Here's how the part is built. I have some questions about the finished solid (model axes, mm). A direction names the side the tool comes from. Coordinates: 2 decimals unless noted, no trailing zeros. Use one line per item in the form item = value. Start each with the question number.
(1) Will these pins go through, and if not, where does the flat tip stop? P1, Ø1.6, axis at x = 78, z = 74.5, coming from the -Y side; P2, Ø1.7, axis at x = 74.5, z = 139, coming from the +Y side; P3, Ø4, axis at y = 20, z = 222.5, coming from the -X side.
(2) Imagine slicing it at A-A, the plane y = 36. State how many separate pieces and enclosed holes the cut face has, and give its area (3 significant figures).
(3) Please list where these lines run through material, in increasing order: L1, parallel to Z at x = 196, y = 20; L2, parallel to Z at x = 45, y = 7; L3, parallel to X at y = 5.75, z = 74.5.
(4) On a 3-axis mill with a long thin cutter (end or side, diameter ignored), from which of +Z, -Z, +X, -X, +Y, -Y can I reach the whole of each face in a straight line? I mean faces 3 (the cylindrical face through (197.29, 17.52, 121.72)), 4 (the flat face through (124, 15, 121)). Say none if no direction works.
(5) Thinking about a two-plate mould opening in X: for faces 1 (the cylindrical face through (197.29, 17.52, 21.72)), 2 (the flat face through (195.455, 29.33, 120.785)), which applies, +X half, -X half, draft (parallel to the pull), parting line (faces both ways), or undercut?
```python
from build123d import *

# Parameters (mm, degrees)
EXTRUDE_1_DEPTH       = 245
EXTRUDE_3_DEPTH       = 245
PATTERN_CURVE_1_COUNT = 19
PATTERN_CURVE_1_PITCH = 9.75
SKETCH_6_R            = 2.5
CUT_EXTRUDE_3_DEPTH   = 8
SKETCH_7_R            = 2.6
CUT_EXTRUDE_4_DEPTH   = 6
SKETCH_8_R            = 4.5
SKETCH_8_R_2          = 3.4
CUT_EXTRUDE_5_DEPTH   = 6
CUT_EXTRUDE_START     = -6
SKETCH_9_R            = 2.6
CUT_EXTRUDE_6_DEPTH   = 6
EXTRUDE_4_REACH       = 321.453
SKETCH_11_R           = 2.6
EXTRUDE_5_REACH       = 321.453
SKETCH_12_R           = 4.5
SKETCH_12_R_2         = 3.4
SKETCH_19_R           = 2.6
CUT_EXTRUDE_12_DEPTH  = 8
SKETCH_21_R           = 2.6
SKETCH_21_R_2         = 1.6
SKETCH_21_R_3         = 1.3
SKETCH_21_R_4         = 2.1
CUT_EXTRUDE_13_DEPTH  = 10


with BuildPart() as part:
    # Эскиз1 → Вытянуть1 (new body)
    with BuildSketch(Plane.XY):
        with BuildLine():
            Line((0, 45), (2.564446908, 45))
            ThreePointArc((2.564446908, 45), (3.247630994, 44.730246195), (3.562232066, 44.066519011))
            Line((3.562232066, 44.066519011), (5.5, 15))
            Line((5.5, 15), (194.5, 15))
            Line((194.5, 15), (196.437767934, 44.066519011))
            ThreePointArc((196.437767934, 44.066519011), (196.752369006, 44.730246195), (197.435553092, 45))
            Line((197.435553092, 45), (200, 45))
            Line((200, 45), (200, 0))
            Line((200, 0), (0, 0))
            Line((0, 0), (0, 45))
        make_face()
    extrude(amount=EXTRUDE_1_DEPTH)

    # Эскиз2 → Вытянуть3 (add)
    with BuildSketch(Plane.XY.offset(245)):
        with BuildLine():
            Line((11.5, 44.5), (10, 15))
            Line((10, 15), (14, 15))
            Line((14, 15), (12.5, 44.5))
            ThreePointArc((12.5, 44.5), (12, 45), (11.5, 44.5))
        make_face()
    extrude_3 = extrude(amount=-EXTRUDE_3_DEPTH)

    # Кривая1: Вытянуть3 ×19
    with Locations(*[(i * PATTERN_CURVE_1_PITCH, 0, 0) for i in range(1, PATTERN_CURVE_1_COUNT)]):
        add(extrude_3)

    # Эскиз6 → Вырез-Вытянуть3 (cut)
    with BuildSketch(Plane(origin=(0, 0, 0), x_dir=(-1, 0, 0), z_dir=(0, 0, -1))):
        with Locations((-4, 6)):
            Circle(SKETCH_6_R)
        with Locations(Location((-196, 6, 0), (0, 0, 180))):
            Circle(SKETCH_6_R)
    extrude(amount=-CUT_EXTRUDE_3_DEPTH, mode=Mode.SUBTRACT)

    # Эскиз7 → Вырез-Вытянуть4 (cut)
    with BuildSketch(Plane.ZY):
        with Locations(Location((22.5, 20, 0), (0, 0, 270))):
            Circle(SKETCH_7_R)
        with Locations(Location((222.5, 20, 0), (0, 0, 270))):
            Circle(SKETCH_7_R)
        with Locations(Location((122.5, 20, 0), (0, 0, 270))):
            Circle(SKETCH_7_R)
    extrude(amount=-CUT_EXTRUDE_4_DEPTH, mode=Mode.SUBTRACT)

    # Эскиз8 → Вырез-Вытянуть5 (cut)
    with BuildSketch(Plane(origin=(200, 0, 0), x_dir=(0, 0, -1), z_dir=(1, 0, 0))):
        with Locations((-80, 30)):
            Circle(SKETCH_8_R)
        with Locations((-165, 30)):
            Circle(SKETCH_8_R_2)
    extrude(amount=-CUT_EXTRUDE_5_DEPTH, mode=Mode.SUBTRACT)

    # Эскиз9 → Вырез-Вытянуть6 (cut)
    with BuildSketch(Plane(origin=(200, 0, 0), x_dir=(0, 0, -1), z_dir=(1, 0, 0)).offset(CUT_EXTRUDE_START)):
        with Locations(Location((-22.5, 20, 0), (0, 0, 270))):
            Circle(SKETCH_9_R)
        with Locations(Location((-122.5, 20, 0), (0, 0, 270))):
            Circle(SKETCH_9_R)
        with Locations(Location((-222.5, 20, 0), (0, 0, 270))):
            Circle(SKETCH_9_R)
    extrude(amount=CUT_EXTRUDE_6_DEPTH, mode=Mode.SUBTRACT)

    # Вытянуть4: up to this face of the body (flat: up to its plane)
    extrude_4_end = Plane(part.part.faces().sort_by_distance((4.525378677, 29.61931985, 122.5))[0])
    # Эскиз11 → Вытянуть4 (add, up to the picked face)
    with BuildSketch(Plane.ZY, mode=Mode.PRIVATE) as extrude_4_sk1:
        with Locations(Location((22.5, 20, 0), (0, 0, 180))):
            Circle(SKETCH_11_R)
    extrude_4_tool1 = split(extrude(extrude_4_sk1.sketch, amount=-EXTRUDE_4_REACH, mode=Mode.PRIVATE), bisect_by=extrude_4_end, keep=Keep.BOTH, mode=Mode.PRIVATE)
    # Эскиз11 → Вытянуть4 (add, up to the picked face)
    with BuildSketch(Plane.ZY, mode=Mode.PRIVATE) as extrude_4_sk2:
        with Locations(Location((122.5, 20, 0), (0, 0, 180))):
            Circle(SKETCH_11_R)
    extrude_4_tool2 = split(extrude(extrude_4_sk2.sketch, amount=-EXTRUDE_4_REACH, mode=Mode.PRIVATE), bisect_by=extrude_4_end, keep=Keep.BOTH, mode=Mode.PRIVATE)
    # Эскиз11 → Вытянуть4 (add, up to the picked face)
    with BuildSketch(Plane.ZY, mode=Mode.PRIVATE) as extrude_4_sk3:
        with Locations(Location((222.5, 20, 0), (0, 0, 180))):
            Circle(SKETCH_11_R)
    extrude_4_tool3 = split(extrude(extrude_4_sk3.sketch, amount=-EXTRUDE_4_REACH, mode=Mode.PRIVATE), bisect_by=extrude_4_end, keep=Keep.BOTH, mode=Mode.PRIVATE)
    add(extrude_4_tool1.solids().sort_by(Axis((0, 20, 22.5), (1, 0, 0)))[0])
    add(extrude_4_tool2.solids().sort_by(Axis((0, 20, 122.5), (1, 0, 0)))[0])
    add(extrude_4_tool3.solids().sort_by(Axis((0, 20, 222.5), (1, 0, 0)))[0])

    # Вытянуть5: up to this face of the body (flat: up to its plane)
    extrude_5_end = Plane(part.part.faces().sort_by_distance((195.474256805, 29.613852069, 122.666761542))[0])
    # Эскиз12 → Вытянуть5 (add, up to the picked face)
    with BuildSketch(Plane(origin=(200, 0, 0), x_dir=(0, 0, -1), z_dir=(1, 0, 0)), mode=Mode.PRIVATE) as extrude_5_sk1:
        with Locations((-80, 30)):
            Circle(SKETCH_12_R)
    extrude_5_tool1 = split(extrude(extrude_5_sk1.sketch, amount=-EXTRUDE_5_REACH, mode=Mode.PRIVATE), bisect_by=extrude_5_end, keep=Keep.BOTH, mode=Mode.PRIVATE)
    # Эскиз12 → Вытянуть5 (add, up to the picked face)
    with BuildSketch(Plane(origin=(200, 0, 0), x_dir=(0, 0, -1), z_dir=(1, 0, 0)), mode=Mode.PRIVATE) as extrude_5_sk2:
        with Locations((-165, 30)):
            Circle(SKETCH_12_R_2)
    extrude_5_tool2 = split(extrude(extrude_5_sk2.sketch, amount=-EXTRUDE_5_REACH, mode=Mode.PRIVATE), bisect_by=extrude_5_end, keep=Keep.BOTH, mode=Mode.PRIVATE)
    add(extrude_5_tool1.solids().sort_by(Axis((200, 30, 80), (-1, 0, 0)))[0])
    add(extrude_5_tool2.solids().sort_by(Axis((200, 30, 165), (-1, 0, 0)))[0])

    # Эскиз19 → Вырез-Вытянуть12 (cut)
    with BuildSketch(Plane.ZY):
        with Locations(Location((222.5, 20, 0), (0, 0, 180))):
            Circle(SKETCH_19_R)
        with Locations(Location((122.5, 20, 0), (0, 0, 180))):
            Circle(SKETCH_19_R)
        with Locations(Location((22.5, 20, 0), (0, 0, 180))):
            Circle(SKETCH_19_R)
    extrude(amount=-CUT_EXTRUDE_12_DEPTH, mode=Mode.SUBTRACT)

    # Эскиз21 → Вырез-Вытянуть13 (cut)
    with BuildSketch(Plane.XZ):
        with Locations((118, 96.5)):
            Circle(SKETCH_21_R)
        with Locations((45, 165)):
            Circle(SKETCH_21_R_2)
        with Locations((45, 15)):
            Circle(SKETCH_21_R_2)
        with Locations((155, 15)):
            Circle(SKETCH_21_R_2)
        with Locations((155, 165)):
            Circle(SKETCH_21_R_2)
        with Locations((78, 74.5)):
            Circle(SKETCH_21_R_3)
        with Locations((123, 74.5)):
            Circle(SKETCH_21_R_3)
        with Locations((78, 45)):
            Circle(SKETCH_21_R_3)
        with Locations((123, 45)):
            Circle(SKETCH_21_R_3)
        with Locations((122.5, 129.25)):
            Circle(SKETCH_21_R_3)
        with Locations((98, 235)):
            Circle(SKETCH_21_R_4)
        with Locations((145, 100)):
            Circle(SKETCH_21_R_4)
        with Locations((98, 180)):
            Circle(SKETCH_21_R_4)
    extrude(amount=-CUT_EXTRUDE_13_DEPTH, mode=Mode.SUBTRACT)


solid = part.part
```
Answer:
q1.P1 = 10
q1.P2 = 15
q1.P3 = 10.15
q2.separate_pieces = 21
q2.enclosed_holes = 0
q2.area = 10,700 mm²
q3.L1 = 0 to 19.9, 25.1 to 119.9, 125.1 to 219.9, 225.1 to 245
q3.L2 = 0 to 13.4, 16.6 to 163.4, 166.6 to 245
q3.L3 = 0 to 76.7, 79.3 to 121.7, 124.3 to 200
q4.face_3 = +X
q4.face_4 = +Z, -Z, +Y
q5.face_1 = draft
q5.face_2 = undercut
